For this review, take the finished solid that the model builds, in its own axes (mm). A direction names the side the tool comes from. Give positions to 0.01 mm unless a question says otherwise; leave off trailing zeros. Write each loop counter-clockwise with the first axis right and the second up, starting at its lowest first coordinate (ties: lowest second). Pieces come first, ordered by that corner, then holes. Notation, with made-up numbers: (62, 31) -> (98, 31) arc R35 cw to (98, 70) -> close; hole circle Ø3 at (-7.5, 72.25). An arc over 180 degrees is marked (long way). Write item = value, one per line.
```python
from build123d import *

# Parameters (mm, degrees)
SKETCH1_W           = 140
SKETCH1_H           = 119
BOSS_EXTRUDE1_DEPTH = 5
FILLET1_R           = 3
SHELL1_START        = -67
SHELL1_OUTLINE_W    = 2
SHELL1_OUTLINE_H    = 113
SHELL1_DEPTH        = 134
FILLET2_R           = 3
CUT_EXTRUDE1_DEPTH  = 1
CUT_EXTRUDE2_DEPTH  = 0.1
FILLET3_R           = 1
FILLET5_R           = 0.5


# Read off the part's stored shape, not the designer's step: Shell1
with BuildPart() as part:
    # Sketch1 → Boss-Extrude1 (new body)
    with BuildSketch(Plane(origin=(0, 0, 0), x_dir=(1, 0, 0), z_dir=(0, 1, 0))):
        Rectangle(SKETCH1_W, SKETCH1_H)
    extrude(amount=BOSS_EXTRUDE1_DEPTH)

    # Fillet1
    fillet1_edges = [part.edges().sort_by_distance(p)[0] for p in [
        (70, 2.5, 59.5),
        (-70, 2.5, 59.5),
        (-70, 2.5, -59.5),
        (70, 2.5, -59.5),
    ]]
    fillet(fillet1_edges, radius=FILLET1_R)

    # Shell1 outline → Shell1 (cut)
    with BuildSketch(Plane.YZ.offset(SHELL1_START)):
        with Locations((1, 0)):
            Rectangle(SHELL1_OUTLINE_W, SHELL1_OUTLINE_H)
    extrude(amount=SHELL1_DEPTH, mode=Mode.SUBTRACT)

    # Fillet2
    fillet2_edges = [part.edges().sort_by_distance(p)[0] for p in [
        (67, 1, -56.5),
        (-67, 1, -56.5),
        (-67, 1, 56.5),
        (67, 1, 56.5),
    ]]
    fillet(fillet2_edges, radius=FILLET2_R)

    # Sketch2 → Cut-Extrude1 (cut)
    with BuildSketch(Plane.XZ):
        with BuildLine():
            Line((68.5, -53.5), (68.5, 53.5))
            ThreePointArc((68.5, 53.5), (67.181980515, 56.681980515), (64, 58))
            Line((64, 58), (-64, 58))
            ThreePointArc((-64, 58), (-67.181980515, 56.681980515), (-68.5, 53.5))
            Line((-68.5, 53.5), (-68.5, -53.5))
            ThreePointArc((-68.5, -53.5), (-67.181980515, -56.681980515), (-64, -58))
            Line((-64, -58), (64, -58))
            ThreePointArc((64, -58), (67.181980515, -56.681980515), (68.5, -53.5))
        make_face()
        with BuildLine():
            Line((67, 53.5), (67, -53.5))
            ThreePointArc((67, -53.5), (66.121320344, -55.621320344), (64, -56.5))
            Line((64, -56.5), (-64, -56.5))
            ThreePointArc((-64, -56.5), (-66.121320344, -55.621320344), (-67, -53.5))
            Line((-67, -53.5), (-67, 53.5))
            ThreePointArc((-67, 53.5), (-66.121320344, 55.621320344), (-64, 56.5))
            Line((-64, 56.5), (64, 56.5))
            ThreePointArc((64, 56.5), (66.121320344, 55.621320344), (67, 53.5))
        make_face(mode=Mode.SUBTRACT)
    extrude(amount=-CUT_EXTRUDE1_DEPTH, mode=Mode.SUBTRACT)

    # Sketch3 → Cut-Extrude2 (cut)
    with BuildSketch(Plane.XZ):
        with BuildLine():
            Line((70, -56.5), (70, 56.5))
            ThreePointArc((70, 56.5), (69.121320344, 58.621320344), (67, 59.5))
            Line((67, 59.5), (-67, 59.5))
            ThreePointArc((-67, 59.5), (-69.121320344, 58.621320344), (-70, 56.5))
            Line((-70, 56.5), (-70, -56.5))
            ThreePointArc((-70, -56.5), (-69.121320344, -58.621320344), (-67, -59.5))
            Line((-67, -59.5), (67, -59.5))
            ThreePointArc((67, -59.5), (69.121320344, -58.621320344), (70, -56.5))
        make_face()
        with BuildLine():
            Line((-64, -58), (64, -58))
            ThreePointArc((64, -58), (67.181980515, -56.681980515), (68.5, -53.5))
            Line((68.5, -53.5), (68.5, 53.5))
            ThreePointArc((68.5, 53.5), (67.181980515, 56.681980515), (64, 58))
            Line((64, 58), (-64, 58))
            ThreePointArc((-64, 58), (-67.181980515, 56.681980515), (-68.5, 53.5))
            Line((-68.5, 53.5), (-68.5, -53.5))
            ThreePointArc((-68.5, -53.5), (-67.181980515, -56.681980515), (-64, -58))
        make_face(mode=Mode.SUBTRACT)
    extrude(amount=-CUT_EXTRUDE2_DEPTH, mode=Mode.SUBTRACT)

    # Fillet3
    fillet3_edges = [part.edges().sort_by_distance(p)[0] for p in [
        (70, 5, 0),
        (0, 5, 59.5),
        (0, 5, -59.5),
        (-70, 5, 0),
        (-69.121320344, 5, 58.621320344),
        (69.121320344, 5, -58.621320344),
        (-69.121320344, 5, -58.621320344),
        (69.121320344, 5, 58.621320344),
    ]]
    fillet(fillet3_edges, radius=FILLET3_R)

    # Fillet5
    fillet5_edges = [part.edges().sort_by_distance(p)[0] for p in [
        (-68.5, 0.1, 0),
        (-67.181980515, 0.1, -56.681980515),
        (0, 0.1, -58),
        (67.181980515, 0.1, -56.681980515),
        (68.5, 0.1, 0),
        (67.181980515, 0.1, 56.681980515),
        (0, 0.1, 58),
        (-67.181980515, 0.1, 56.681980515),
        (-67, 1, 0),
        (-66.121320344, 1, -55.621320344),
        (0, 1, -56.5),
        (66.121320344, 1, -55.621320344),
        (67, 1, 0),
        (66.121320344, 1, 55.621320344),
        (0, 1, 56.5),
        (-66.121320344, 1, 55.621320344),
    ]]
    fillet(fillet5_edges, radius=FILLET5_R)


solid = part.part
```
(1) Take a section at A-A (x = 8.5). Write out the cut boundary in (y, z), plus the area to 3 significant figures.
Answers below:
outline = (0.1, -59.5) -> (4, -59.5) arc R1 ccw to (5, -58.5) -> (5, 58.5) arc R1 ccw to (4, 59.5) -> (0.1, 59.5) -> (0.1, 58.5) arc R0.5 ccw to (0.6, 58) -> (1, 58) -> (1, 57) arc R0.5 ccw to (1.5, 56.5) -> (2, 56.5) -> (2, -56.5) -> (1.5, -56.5) arc R0.5 ccw to (1, -57) -> (1, -58) -> (0.6, -58) arc R0.5 ccw to (0.1, -58.5) -> close
area = 365 mm^2
(2) To check wall thickness, follow probe 1 along Z at (x, y) = (52, 0.6); probe 2 along X at (y, z) = (0.55, 29.5); probe 3 along Z at (x, y) = (-49, 1.85). State the ranges of each line that lie inside material, in increasing order.
Answers below:
probe_1 = -59.5 to -58, 58 to 59.5
probe_2 = -70 to -68.5, 68.5 to 70
probe_3 = -59.5 to -56.5, 56.5 to 59.5
(3) Tool access review of faces 1 (the face through (-1, 2, -1)), 2 (the face through (-1, 5, -1)): name each direction out of +Z, -Z, +X, -X, +Y, -Y from which nothing blocks a thin tool from reaching the whole face with its end or side.
Answers below:
face_1 = -Y
face_2 = +Z, -Z, +X, -X, +Y
(4) For pin 1 (10 mm diameter, centred on x = -38.5, z = 40.5, fed in from -Y), flat-tipped, find the tip position at first contact; note if it passes through.
Answers below:
pin_1 = 2
(5) The part is to be moulded in two halves that separate along X. For faces 3 (the face through (66.1, 1.75, 55.64)), 4 (the face through (-1, 2, 59.5)), 5 (the face through (-69.14, 2.08, 58.6)), say which applies: released by +X, released by -X, zero draft, split by the parting line, or undercut.
Answers below:
face_3 = undercut
face_4 = zero draft
face_5 = released by -X
(6) Take a section at B-B (z = 8). Write out the cut boundary in (x, y), plus the area to 3 significant figures.
Answers below:
outline = (-70, 0.1) -> (-69, 0.1) arc R0.5 ccw to (-68.5, 0.6) -> (-68.5, 1) -> (-67.5, 1) arc R0.5 ccw to (-67, 1.5) -> (-67, 2) -> (67, 2) -> (67, 1.5) arc R0.5 ccw to (67.5, 1) -> (68.5, 1) -> (68.5, 0.6) arc R0.5 ccw to (69, 0.1) -> (70, 0.1) -> (70, 4) arc R1 ccw to (69, 5) -> (-69, 5) arc R1 ccw to (-70, 4) -> close
area = 428 mm^2
